from build123d import *

# Parameters (mm, degrees)
SKETCH1_R           = 3.5
BOSS_EXTRUDE1_DEPTH = 2


with BuildPart() as part:
    # Sketch1 → Boss-Extrude1 (new body)
    with BuildSketch(Plane(origin=(0, 0, 0), x_dir=(1, 0, 0), z_dir=(0, 1, 0))):
        with BuildLine():
            Line((0, 5), (0, 67.928932188))
            ThreePointArc((0, 67.928932188), (3.086582838, 72.548329851), (8.535533906, 71.464466094))
            Line((8.535533906, 71.464466094), (17.071067812, 62.928932188))
            ThreePointArc((17.071067812, 62.928932188), (19.238795325, 59.6846987), (20, 55.857864376))
            Line((20, 55.857864376), (20, 30))
            ThreePointArc((20, 30), (22.928932188, 22.928932188), (30, 20))
            Line((30, 20), (55.857864376, 20))
            ThreePointArc((55.857864376, 20), (59.6846987, 19.238795325), (62.928932188, 17.071067812))
            Line((62.928932188, 17.071067812), (71.464466094, 8.535533906))
            ThreePointArc((71.464466094, 8.535533906), (72.548329851, 3.086582838), (67.928932188, 0))
            Line((67.928932188, 0), (5, 0))
            ThreePointArc((5, 0), (1.464466094, 1.464466094), (0, 5))
        make_face()
        with Locations(Location((10, 60, 0), (0, 0, 270))):
            Circle(SKETCH1_R, mode=Mode.SUBTRACT)
        with Locations(Location((10, 35, 0), (0, 0, 270))):
            Circle(SKETCH1_R, mode=Mode.SUBTRACT)
        with Locations(Location((35, 10, 0), (0, 0, 270))):
            Circle(SKETCH1_R, mode=Mode.SUBTRACT)
        with Locations(Location((60, 10, 0), (0, 0, 270))):
            Circle(SKETCH1_R, mode=Mode.SUBTRACT)
    extrude(amount=BOSS_EXTRUDE1_DEPTH)


solid = part.part
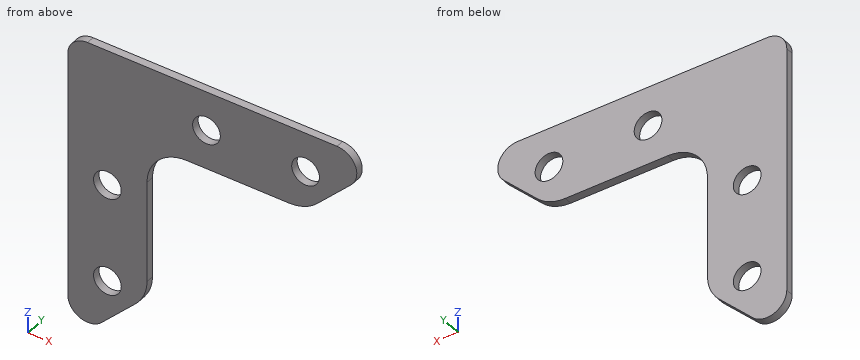
Verification items for the finished model (mm, model axes). Give positions to 0.01 mm unless a question says otherwise; leave off trailing zeros. Loops run counter-clockwise (first coordinate to the right, second up) from the corner with the lowest first, then second, coordinate; pieces in that order, holes last.
1. Cross-section at B-B on y = 1.6. Record the cut outline in (x, z), and give its area (3 significant figures).
Derived:
outline: (0, -67.93) arc R5 ccw to (8.54, -71.46) - (17.07, -62.93) arc R10 ccw to (20, -55.86) - (20, -30) arc R10 cw to (30, -20) - (55.86, -20) arc R10 ccw to (62.93, -17.07) - (71.46, -8.54) arc R5 ccw to (67.93, 0) - (5, 0) arc R5 ccw to (0, -5) - close; hole circle Ø7 at (10, -60); hole circle Ø7 at (10, -35); hole circle Ø7 at (35, -10); hole circle Ø7 at (60, -10)
area: 2,200 mm2
2. Cross-section at C-C on x = 35. Record the cut outline in (y, z), and give its area (3 significant figures).
Derived:
outline: (0, -20) - (2, -20) - (2, -13.5) - (0, -13.5) - close; (0, -6.5) - (2, -6.5) - (2, 0) - (0, 0) - close
area: 26.0 mm2
3. Cross-section at A-A on z = -10. Record the cut outline in (x, y).
Derived:
outline: (0, 0) - (31.5, 0) - (31.5, 2) - (0, 2) - close; (38.5, 0) - (56.5, 0) - (56.5, 2) - (38.5, 2) - close; (63.5, 0) - (70, 0) - (70, 2) - (63.5, 2) - close
4. Material ranges on probe 1 along X at (y, z) = (1.15, -35); probe 2 along X at (y, z) = (0.7, -49); probe 3 along Z at (x, y) = (53, 1.1), recorded low to high.
Derived:
probe 1: x = 0 to 6.5, 13.5 to 20
probe 2: x = 0 to 20
probe 3: z = -20 to 0
5. Go/stop test with a flat-tipped pin: P1, Ø5.5, axis at x = 35, z = -10, coming from the +Y side. Record where the tip stops, or that it passes through.
Derived:
P1: passes through
6. Cross-section at D-D on z = -35. Record the cut outline in (x, y).
Derived:
outline: (0, 0) - (6.5, 0) - (6.5, 2) - (0, 2) - close; (13.5, 0) - (20, 0) - (20, 2) - (13.5, 2) - close
